from build123d import *

# Parameters (mm, degrees)
SKETCH1_W           = 8
SKETCH1_H           = 4
BOSS_EXTRUDE1_DEPTH = 0.2
FILLET1_R           = 1
BOSS_EXTRUDE2_DEPTH = 0.2
SKETCH3_W           = 3.5
SKETCH3_H           = 2.65
BOSS_EXTRUDE3_DEPTH = 0.98


with BuildPart() as part:
    # Sketch1 → Boss-Extrude1 (new body)
    with BuildSketch(Plane(origin=(0, 0, 0), x_dir=(1, 0, 0), z_dir=(0, 1, 0))):
        Rectangle(SKETCH1_W, SKETCH1_H)
    extrude(amount=BOSS_EXTRUDE1_DEPTH)

    # Fillet1
    fillet1_edges = [part.edges().sort_by_distance(p)[0] for p in [
        (4, 0.1, 2),
        (-4, 0.1, 2),
        (-4, 0.1, -2),
        (4, 0.1, -2),
    ]]
    fillet(fillet1_edges, radius=FILLET1_R)

    # Sketch2 → Boss-Extrude2 (add)
    with BuildSketch(Plane(origin=(0, 0.2, 0), x_dir=(1, 0, 0), z_dir=(0, 1, 0))):
        Polygon((4, 0.2), (4, 0), (4.6, 0), (4.6, 1), (5.2, 1), (5.2, -1), (5.8, -1), (5.8, 1), (6.4, 1), (6.4, -1), (7, -1), (7, 0), (7.6, 0), (7.6, 0.2), (6.8, 0.2), (6.8, -0.8), (6.6, -0.8), (6.6, 1.2), (5.6, 1.2), (5.6, -0.8), (5.4, -0.8), (5.4, 1.2), (4.4, 1.2), (4.4, 0.2), align=None)
        Polygon((4.6, 0), (4, 0), (4, -0.2), (4.8, -0.2), (4.8, 0.8), (5, 0.8), (5, -1.2), (6, -1.2), (6, 0.8), (6.2, 0.8), (6.2, -1.2), (7.2, -1.2), (7.2, -0.2), (7.6, -0.2), (7.6, 0), (7, 0), (7, -1), (6.4, -1), (6.4, 1), (5.8, 1), (5.8, -1), (5.2, -1), (5.2, 1), (4.6, 1), align=None)
    boss_extrude2 = extrude(amount=-BOSS_EXTRUDE2_DEPTH)

    # Mirror1: Boss-Extrude2 across plane
    add(boss_extrude2.mirror(Plane(origin=(0, 0, 0), x_dir=(0, 0, 1), z_dir=(1, 0, 0))))

    # Sketch3 → Boss-Extrude3 (add)
    with BuildSketch(Plane(origin=(0, 0.2, 0), x_dir=(1, 0, 0), z_dir=(0, 1, 0))):
        Rectangle(SKETCH3_W, SKETCH3_H)
    extrude(amount=BOSS_EXTRUDE3_DEPTH)


solid = part.part
Input: part model. Units: mm. Frame: model coordinates. A direction names the side the tool comes from. Coordinates: 2 decimals unless noted, no trailing zeros. Loops run counter-clockwise (first coordinate to the right, second up) from the corner with the lowest first, then second, coordinate; pieces in that order, holes last. Notation, with made-up numbers: (-39.5, 89.25) -> (-2.5, 89.25) arc R16 ccw to (-2.5, 95.25) -> close; hole circle Ø1 at (-18, -20.5). An arc over 180 degrees is marked (long way). Write item = value, one per line. Start each with the question number.
Item 1: Cut plane B-B, the plane y = 0.95. Return loops of the section in (x, z) (3 decimals), plus the area to 4 significant figures.
Item 2: Cut plane A-A, the plane x = -1. Return loops of the section in (y, z) (3 decimals), plus the area to 3 significant figures.
Item 3: Cut plane C-C, the plane x = -5.25. Return loops of the section in (y, z), plus the area to 3 significant figures.
Item 4: Reachability of faces 1 (the face through (0, 1, 1.325)), 2 (the face through (-1.75, 1, 0)), 3 (the face through (0, 1, -1.325)), 4 (the face through (1.75, 1, 0)) from +Z, -Z, +X, -X, +Y, -Y: full face, straight path, thin tool, end or side. Return the list, or none.
Item 5: Material intervals for line 1 (X direction, y = 0.9, z = -0.95); line 2 (Z direction, x = 0.75, y = 1.1) (3 decimals); line 3 (Y direction, x = 3.5, z = -1.2), sorted ascending.
Ans:
q1.outline = (-1.75, -1.325) -> (1.75, -1.325) -> (1.75, 1.325) -> (-1.75, 1.325) -> close
q1.area = 9.275 mm²
q2.outline = (0, -2) -> (0.2, -2) -> (0.2, -1.325) -> (1.18, -1.325) -> (1.18, 1.325) -> (0.2, 1.325) -> (0.2, 2) -> (0, 2) -> close
q2.area = 3.40 mm²
q3.outline = (0, -1.2) -> (0.2, -1.2) -> (0.2, 1.2) -> (0, 1.2) -> close
q3.area = 0.480 mm²
q4.face_1 = +Z, +X, -X, +Y
q4.face_2 = +Z, -Z, -X, +Y
q4.face_3 = -Z, +X, -X, +Y
q4.face_4 = +Z, -Z, +X, +Y
q5.line_1 = -1.75 to 1.75
q5.line_2 = -1.325 to 1.325
q5.line_3 = 0 to 0.2
